Input: dimensioned drawing with shaded views. Units: mm. Origin: part minimum x, y, z. Give positions to 0.01 mm unless a question says otherwise; leave off trailing zeros. Loops run counter-clockwise (first coordinate to the right, second up) from the corner with the lowest first, then second, coordinate; pieces in that order, holes last. Notation, with made-up numbers: M -26,1.5 L 12,1.5 A16 cw 12,16.5 Z; hole C 80.25,79.25 d5. An arc over 180 degrees is marked long. Answer in a Markdown table with one row per item.
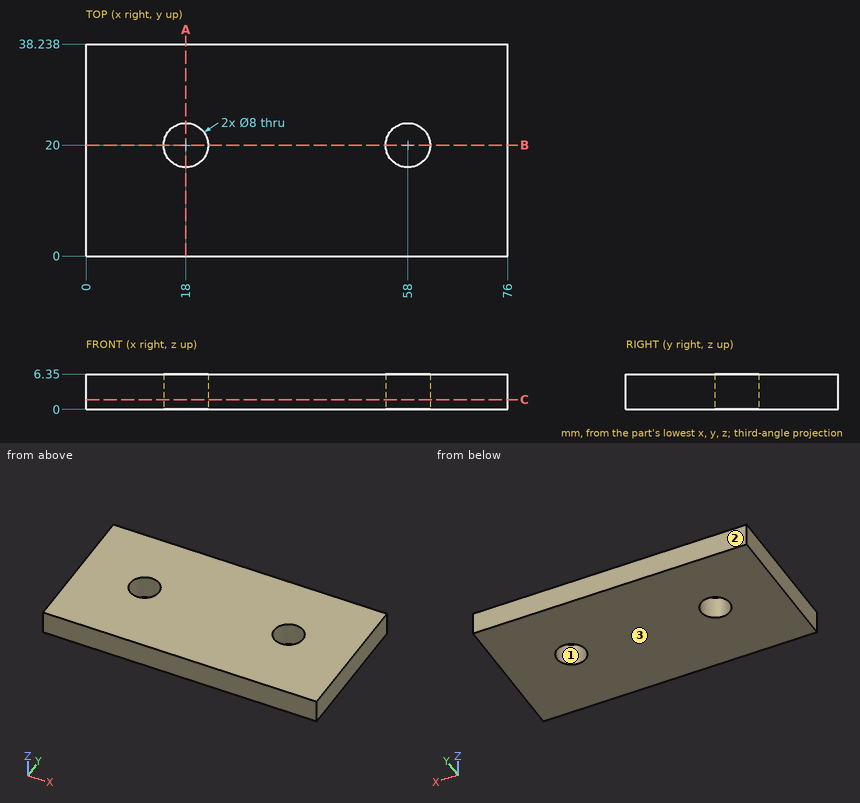
Q1. Mould query, pull axis Y, two halves, no side actions, for the marked faces 1, 2 and 3. Classes: +Y half, -Y half, draft (parallel to the pull), parting line (faces both ways), or undercut.
Values follow:
| item | result |
|---|---|
| face 1 | undercut |
| face 2 | +Y half |
| face 3 | draft |
Q2. Ray query, probe 1 along X at (y, z) = (22.5, 2); probe 2 along Y at (x, z) = (18, 5); probe 3 along X at (y, z) = (19, 1.5). Return the intervals inside material, ascending. Write a range as from..to.
Values follow:
| item | result |
|---|---|
| probe 1 | 0..14.88, 21.12..54.88, 61.12..76 |
| probe 2 | 0..16, 24..38.24 |
| probe 3 | 0..14.13, 21.87..54.13, 61.87..76 |
Q3. Section query A-A (x = 18). Output: boundary loops of the cut face in (y, z).
Values follow:
| item | result |
|---|---|
| outline | M 0,0 L 16,0 L 16,6.35 L 0,6.35 Z; M 24,0 L 38.24,0 L 38.24,6.35 L 24,6.35 Z |
Q4. Section query C-C (z = 1.75). Output: boundary loops of the cut face in (x, y).
Values follow:
| item | result |
|---|---|
| outline | M 0,0 L 76,0 L 76,38.24 L 0,38.24 Z; hole C 18,20 d8; hole C 58,20 d8 |
Q5. Section query B-B (y = 20). Output: boundary loops of the cut face in (x, z), plus the area to 3 significant figures.
Values follow:
| item | result |
|---|---|
| outline | M 0,0 L 14,0 L 14,6.35 L 0,6.35 Z; M 22,0 L 54,0 L 54,6.35 L 22,6.35 Z; M 62,0 L 76,0 L 76,6.35 L 62,6.35 Z |
| area | 381 mm^2 |
